The figure shows three views and two pictorial views of one solid part (mm, origin at its lowest corner). Answer the questions. A direction names the side the tool comes from. Coordinates: 2 decimals unless noted, no trailing zeros. Order: outer loops, then holes, each group sorted by start corner. A loop starts at its lowest first (then second) coordinate and runs counter-clockwise, first axis right, second up.
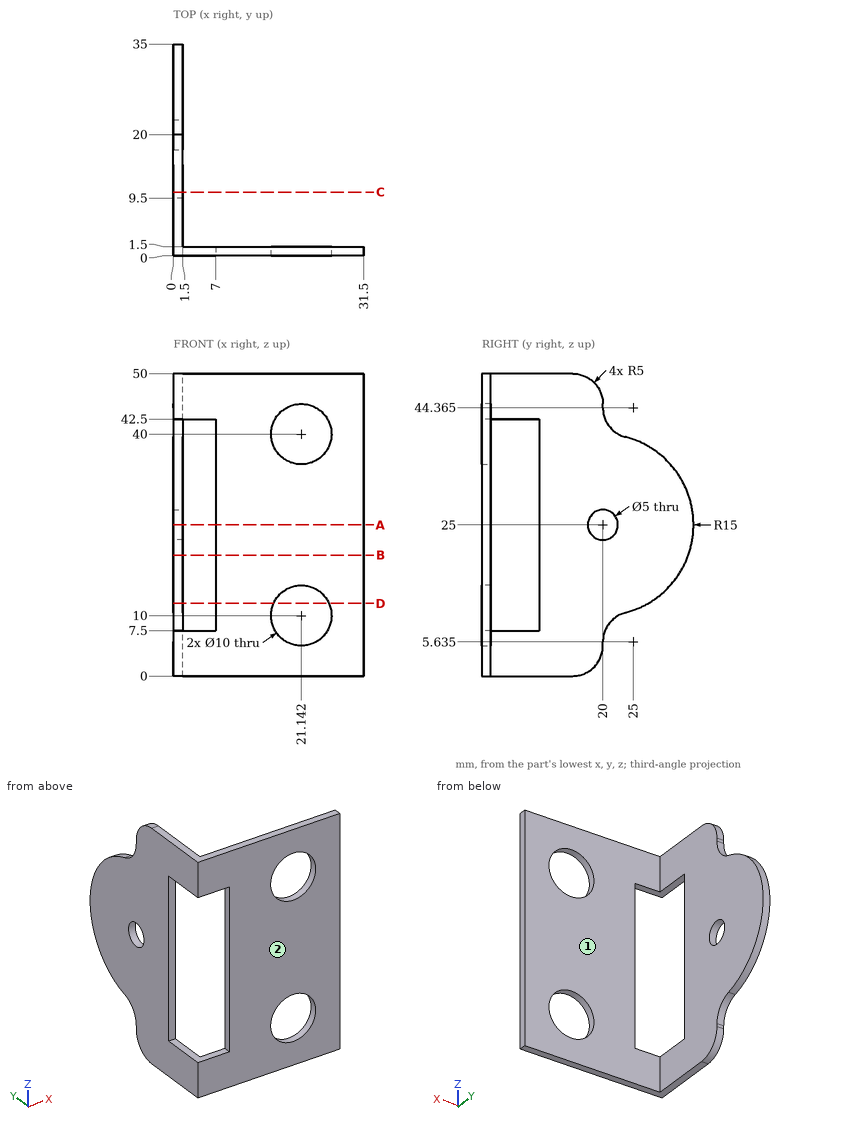
1) Straight lines are drawn through the part: probe 1 along X at (y, z) = (1.1, 40); probe 2 along Y at (x, z) = (17, 7). For each, find the intervals that lie inside material, in ascending order.
2) For the marked faces 1 and 2, determine the directions among +Z, -Z, +X, -X, +Y, -Y from which every point of the face is accessible in a straight line to the end or side of a thin tool.
3) A cutting plane is placed at A-A, the plane z = 25. Write down the section's boundary in (x, y).
4) Each of these flat-tipped pins is pushed along its axis until it touches: P1, Ø12, axis at y = 15, z = 32.5, coming from the -X side; P2, Ø0.8, axis at y = 0.5, z = 19, coming from the -X side; P3, Ø0.5, axis at x = 1, z = 45, coming from the +Y side; P4, Ø12, axis at y = 30.5, z = 8.5, coming from the +X side. Where does it stop, or does it pass through?
5) A cutting plane is placed at D-D, the plane z = 12. Write down the section's boundary in (x, y) (1 decimal).
6) A cutting plane is placed at C-C, the plane y = 10.5. Write down the section's boundary in (x, z).
7) A cutting plane is placed at B-B, the plane z = 20. Write down the section's boundary in (x, y).
Working result:
1. probe 1: x = 7 to 16.14, 26.14 to 31.5
1. probe 2: y = 0 to 1.5
2. face 1: +Z, -Z, +X, +Y
2. face 2: +Z, -Z, +X, -X, -Y
3. outline: (0, 9.5) - (1.5, 9.5) - (1.5, 17.5) - (0, 17.5) - close; (0, 22.5) - (1.5, 22.5) - (1.5, 35) - (0, 35) - close; (7, 0) - (31.5, 0) - (31.5, 1.5) - (7, 1.5) - close
4. P1: stops at x = 0
4. P2: stops at x = 7
4. P3: stops at y = 20
4. P4: stops at x = 1.5
5. outline: (0, 9.5) - (1.5, 9.5) - (1.5, 27.5) - (0, 27.5) - close; (7, 0) - (16.6, 0) - (16.6, 1.5) - (7, 1.5) - close; (25.7, 0) - (31.5, 0) - (31.5, 1.5) - (25.7, 1.5) - close
6. outline: (0, 0) - (1.5, 0) - (1.5, 50) - (0, 50) - close
7. outline: (0, 9.5) - (1.5, 9.5) - (1.5, 34.14) - (0, 34.14) - close; (7, 0) - (31.5, 0) - (31.5, 1.5) - (7, 1.5) - close
